Could you check a few things on this model? Use its own coordinates, in mm. Give positions to 0.01 mm unless a question says otherwise; leave off trailing zeros. Loops run counter-clockwise (first coordinate to the right, second up) from the corner with the lowest first, then second, coordinate; pieces in that order, holes last.
1. Imagine slicing it at B-B (z = 2.5). List the corners of the cut face in (x, y) for me.
2. For P1, Ø1.6, axis at x = 25, y = 0, coming from the +Z side; P2, Ø1, axis at y = 1.5, z = 2, coming from the -X side, each with a flat end and sliding along its axis, tell me the tip position at first contact or that it passes through.
3. I need wall thicknesses on line 1 along Y through (x, z) = (0, 2.1); line 2 along X through (y, z) = (0.2, 0.5); line 3 along X through (y, z) = (1.6, 3.45). Which ranges of each line are inside material? Lowest first, please.
4. Imagine slicing it at A-A (y = 0). List the corners of the cut face in (x, z) for me.
5. Thinking about a two-plate mould opening in X: for faces 1 (the flat face through (13, -2.3, 2)), 2 (the cylindrical face through (-2.3, -0.05, 1.87)), 3 (the cylindrical face through (0, 1, 2)), which applies, +X half, -X half, draft (parallel to the pull), parting line (faces both ways), or undercut?
6. Imagine slicing it at C-C (y = 1.85). List the corners of the cut face in (x, z) for me, plus the area to 3 significant figures.
```python
from build123d import *

# Parameters (mm, degrees)
SKETCH1_R           = 1
BOSS_EXTRUDE1_DEPTH = 3.8


with BuildPart() as part:
    # Sketch1 → Boss-Extrude1 (new body)
    with BuildSketch(Plane.XY):
        with BuildLine():
            Line((0, 2.3), (25, 2.3))
            ThreePointArc((25, 2.3), (27.3, 0), (25, -2.3))
            Line((25, -2.3), (0, -2.3))
            ThreePointArc((0, -2.3), (-2.3, 0), (0, 2.3))
        make_face()
        with Locations(Location((0, 0, 0), (0, 0, 180))):
            Circle(SKETCH1_R, mode=Mode.SUBTRACT)
        with Locations(Location((25, 0, 0), (0, 0, 180))):
            Circle(SKETCH1_R, mode=Mode.SUBTRACT)
    extrude(amount=BOSS_EXTRUDE1_DEPTH)


solid = part.part
```
Derived:
1. outline: (0, -2.3) - (25, -2.3) arc R2.3 ccw to (25, 2.3) - (0, 2.3) arc R2.3 ccw to start; hole circle Ø2 at (0, 0); hole circle Ø2 at (25, 0)
2. P1: passes through
2. P2: stops at x = -2.07
3. line 1: y = -2.3 to -1, 1 to 2.3
3. line 2: x = -2.29 to -0.98, 0.98 to 24.02, 25.98 to 27.29
3. line 3: x = -1.65 to 26.65
4. outline: (-2.3, 0) - (-1, 0) - (-1, 3.8) - (-2.3, 3.8) - close; (1, 0) - (24, 0) - (24, 3.8) - (1, 3.8) - close; (26, 0) - (27.3, 0) - (27.3, 3.8) - (26, 3.8) - close
5. face 1: draft
5. face 2: -X half
5. face 3: undercut
6. outline: (-1.37, 0) - (26.37, 0) - (26.37, 3.8) - (-1.37, 3.8) - close
6. area: 105 mm2
